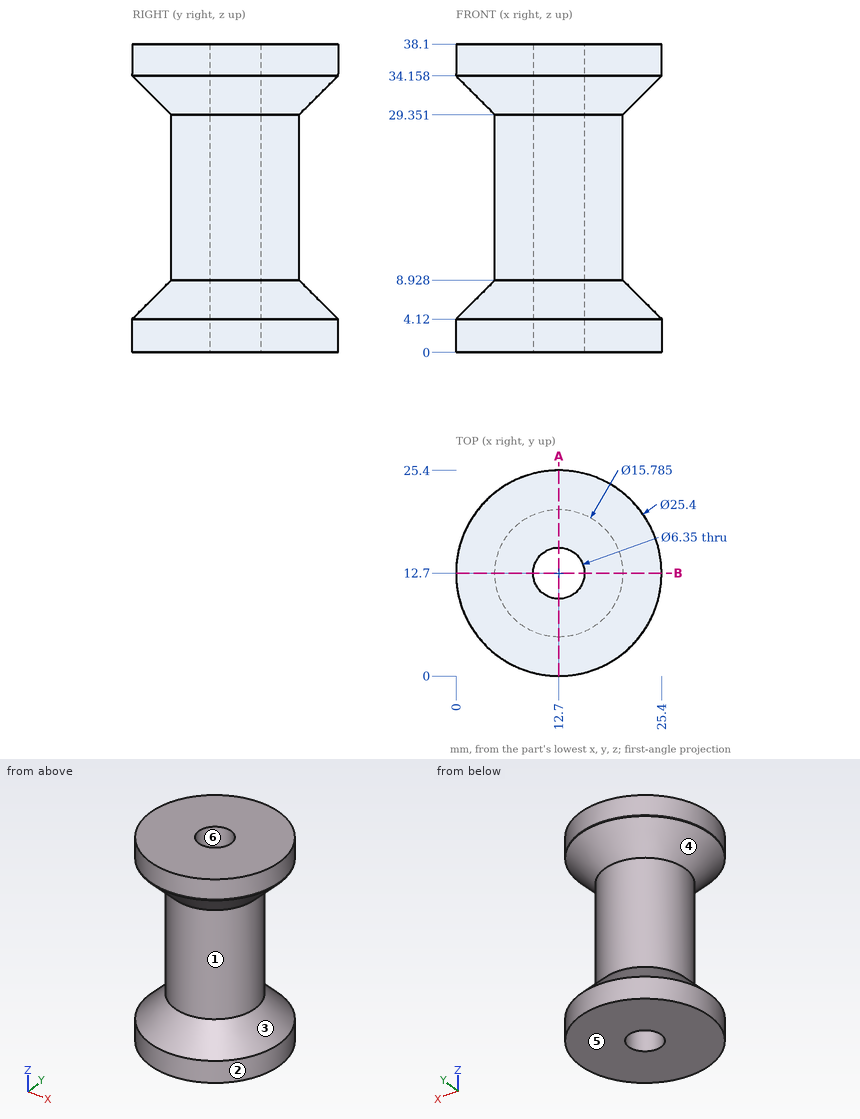
Input: dimensioned drawing with shaded views. Units: mm. Origin: part minimum x, y, z. A direction names the side the tool comes from. Give positions to 0.01 mm unless a question says otherwise; leave off trailing zeros. Write each loop counter-clockwise with the first axis right and the second up, starting at its lowest first coordinate (ties: lowest second). Pieces come first, ordered by that corner, then holes. Notation, with made-up numbers: (54, 78.25) - (98, 78.25) arc R18 cw to (98, 113.25) - close; hole circle Ø3 at (3, 42.5). An arc over 180 degrees is marked (long way). One line per item, written item: value. Start each with the question number.
Q1. Set-up query: the marked faces 1 and 2. Return all of +Z, -Z, +X, -X, +Y, -Y with unobstructed straight access to the full face (end or side cutting, diameter ignored); none if empty.
Q2. First-contact query: pin 1 Ø4 at (x, z) = (15.5, 22.5) entering from -Y; pin 2 Ø2 at (y, z) = (19.5, 10) entering from +X; pin 3 Ø3 at (y, z) = (13.5, 17) entering from -X. Flat tips, straight axial feed; report the tip coordinate or a pass-through.
Q3. Material intervals for probe 1 along Y at (x, z) = (12.7, 17) (1 decimal); probe 2 along Y at (x, z) = (12.7, 29.5) (1 decimal); probe 3 along Z at (x, y) = (1.5, 8) (1 decimal), sorted ascending. Write a range as from..to.
Q4. Draft query along Z for the marked faces 3, 4, 5 and 6. Return one class per face: +Z half, -Z half, draft (parallel to the pull), parting line (faces both ways), or undercut.
Q5. Section query A-A, the plane x = 12.7. Return the cut outline in (y, z) (1 decimal).
Answer:
1. face 1: none
1. face 2: +Z, -Z
2. pin 1: stops at y = 4.85
2. pin 2: stops at x = 18.05
2. pin 3: stops at x = 4.81
3. probe 1: y = 4.8..9.5, 15.9..20.6
3. probe 2: y = 4.7..9.5, 15.9..20.7
3. probe 3: z = 0..4.7, 33.6..38.1
4. face 3: undercut
4. face 4: undercut
4. face 5: -Z half
4. face 6: draft
5. outline: (0, 0) - (9.5, 0) - (9.5, 38.1) - (0, 38.1) - (0, 34.2) - (4.8, 29.4) - (4.8, 8.9) - (0, 4.1) - close; (15.9, 0) - (25.4, 0) - (25.4, 4.1) - (20.6, 8.9) - (20.6, 29.4) - (25.4, 34.2) - (25.4, 38.1) - (15.9, 38.1) - close
